Drawing for the job (mm, zero at the part's lowest x, y, z). Give positions to 0.01 mm unless a question says otherwise; leave off trailing zeros. Order: outer loops, then holes, each group sorted by start corner. A loop starts at its lowest first (then second) coordinate and runs counter-clockwise, first axis right, second up. Notation, with made-up numbers: (-14, 67.5) - (30, 67.5) arc R27 cw to (30, 102.5) - close; hole circle Ø10 at (-0.5, -6). An arc over 180 degrees is marked (long way). One line per item, written item: value.
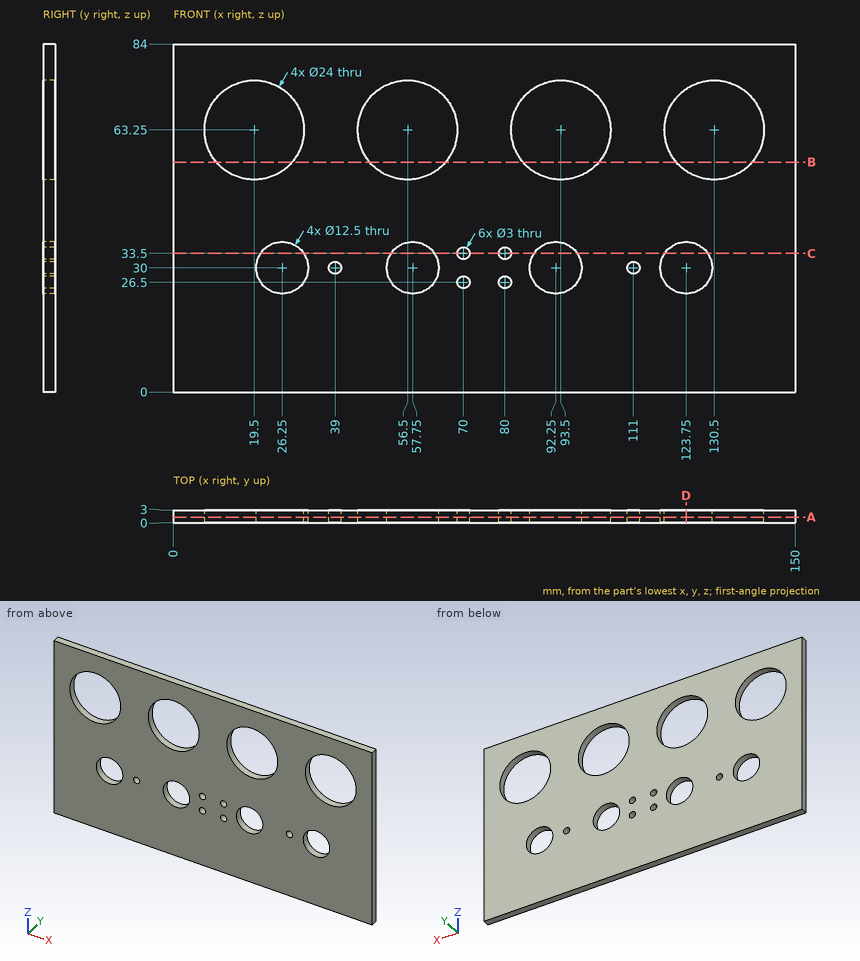
1) Cut at A-A, the plane y = 1.3. Give the number of separate pieces and of enclosed holes in the cut face, then the cut area to 3 significant figures.
Outcome:
separate pieces: 1
enclosed holes: 14
area: 10,300 mm^2
2) Cut at C-C, the plane z = 33.5. Give the cut face in (x, y), then the cut area to 3 significant figures.
Outcome:
outline: (0, 0) - (21.07, 0) - (21.07, 3) - (0, 3) - close; (31.43, 0) - (52.57, 0) - (52.57, 3) - (31.43, 3) - close; (62.93, 0) - (68.5, 0) - (68.5, 3) - (62.93, 3) - close; (71.5, 0) - (78.5, 0) - (78.5, 3) - (71.5, 3) - close; (81.5, 0) - (87.07, 0) - (87.07, 3) - (81.5, 3) - close; (97.43, 0) - (118.57, 0) - (118.57, 3) - (97.43, 3) - close; (128.93, 0) - (150, 0) - (150, 3) - (128.93, 3) - close
area: 308 mm^2
3) Drill centre lines: line 1 along Z through (x, y) = (70.5, 0.1); line 2 along Z through (x, y) = (123.75, 1.05); line 3 along Z through (x, y) = (111, 2.4). Where is each one in solid material? Low to high. Write a range as from..to.
Outcome:
line 1: z = 0..25.09, 27.91..32.09, 34.91..84
line 2: z = 0..23.75, 36.25..53.33, 73.17..84
line 3: z = 0..28.5, 31.5..84
4) Cut at D-D, the plane x = 123.75. Give the cut face in (y, z).
Outcome:
outline: (0, 0) - (3, 0) - (3, 23.75) - (0, 23.75) - close; (0, 36.25) - (3, 36.25) - (3, 53.33) - (0, 53.33) - close; (0, 73.17) - (3, 73.17) - (3, 84) - (0, 84) - close
5) Cut at B-B, the plane z = 55.5. Give the cut face in (x, y), then the cut area to 3 significant figures.
Outcome:
outline: (0, 0) - (10.34, 0) - (10.34, 3) - (0, 3) - close; (28.66, 0) - (47.34, 0) - (47.34, 3) - (28.66, 3) - close; (65.66, 0) - (84.34, 0) - (84.34, 3) - (65.66, 3) - close; (102.66, 0) - (121.34, 0) - (121.34, 3) - (102.66, 3) - close; (139.66, 0) - (150, 0) - (150, 3) - (139.66, 3) - close
area: 230 mm^2
